```python
from build123d import *

# Parameters (mm, degrees)
ESBO_O1_W                  = 42.2
ESBO_O1_H                  = 42.2
RESSALTO_EXTRUS_O1_DEPTH   = 16
CHANFRO4_SIZE              = 7
FILETE3_R                  = 4
ESBO_O2_W                  = 42.3
ESBO_O2_H                  = 42.3
RESSALTO_EXTRUS_O2_DEPTH   = 8
CHANFRO5_SIZE              = 7
FILETE4_R                  = 4
CHANFRO5_OF_ESPELHAR1_SIZE = 7
FILETE4_OF_ESPELHAR1_R     = 4
ESBO_O3_R                  = 11
ESBO_O3_R_2                = 3.5
RESSALTO_EXTRUS_O3_DEPTH   = 2
FILETE5_R                  = 0.5
FILETE6_R                  = 1
ESBO_O4_R                  = 1.5
CORTE_EXTRUS_O1_DEPTH      = 10
PADR_OCIRCULAR1_COUNT      = 4
ESBO_O5_R                  = 2.5
RESSALTO_EXTRUS_O4_DEPTH   = 4
RESSALTO_EXTRUS_O5_DEPTH   = 19
CHANFRO3_SIZE              = 0.5
FILETE2_R                  = 0.5


with BuildPart() as part:
    # Esboço1 → Ressalto-extrusão1 (new, symmetric)
    with BuildSketch(Plane(origin=(0, 0, 0), x_dir=(1, 0, 0), z_dir=(0, 1, 0))):
        Rectangle(ESBO_O1_W, ESBO_O1_H)
    extrude(amount=RESSALTO_EXTRUS_O1_DEPTH, both=True)

    # Chanfro4
    chanfro4_edges = [part.edges().sort_by_distance(p)[0] for p in [
        (21.1, 0, 21.1),
        (-21.1, 0, 21.1),
        (-21.1, 0, -21.1),
        (21.1, 0, -21.1),
    ]]
    chamfer(chanfro4_edges, length=CHANFRO4_SIZE)

    # Filete3
    filete3_edges = [part.edges().sort_by_distance(p)[0] for p in [
        (14.1, 0, 21.1),
        (-14.1, 0, 21.1),
        (-21.1, 0, -14.1),
        (-21.1, 0, 14.1),
        (14.1, 0, -21.1),
        (-14.1, 0, -21.1),
        (21.1, 0, 14.1),
        (21.1, 0, -14.1),
    ]]
    fillet(filete3_edges, radius=FILETE3_R)

    # Esboço2 → Ressalto-extrusão2 (add)
    with BuildSketch(Plane(origin=(0, 16, 0), x_dir=(1, 0, 0), z_dir=(0, 1, 0))):
        Rectangle(ESBO_O2_W, ESBO_O2_H)
    ressalto_extrus_o2 = extrude(amount=RESSALTO_EXTRUS_O2_DEPTH)

    # Chanfro5
    chanfro5_edges = [part.edges().sort_by_distance(p)[0] for p in [
        (21.15, 20, 21.15),
        (21.15, 20, -21.15),
        (-21.15, 20, -21.15),
        (-21.15, 20, 21.15),
    ]]
    chamfer(chanfro5_edges, length=CHANFRO5_SIZE)

    # Filete4
    filete4_edges = [part.edges().sort_by_distance(p)[0] for p in [
        (-14.15, 20, -21.15),
        (14.15, 20, -21.15),
        (21.15, 20, 14.15),
        (21.15, 20, -14.15),
        (-14.15, 20, 21.15),
        (14.15, 20, 21.15),
        (-21.15, 20, -14.15),
        (-21.15, 20, 14.15),
    ]]
    fillet(filete4_edges, radius=FILETE4_R)

    # Espelhar1: Ressalto-extrusão2 across plane
    add(ressalto_extrus_o2.mirror(Plane.ZX))

    # Chanfro5 of Espelhar1
    chanfro5_of_espelhar1_edges = [part.edges().sort_by_distance(p)[0] for p in [
        (21.15, -20, 21.15),
        (21.15, -20, -21.15),
        (-21.15, -20, -21.15),
        (-21.15, -20, 21.15),
    ]]
    chamfer(chanfro5_of_espelhar1_edges, length=CHANFRO5_OF_ESPELHAR1_SIZE)

    # Filete4 of Espelhar1
    filete4_of_espelhar1_edges = [part.edges().sort_by_distance(p)[0] for p in [
        (-14.15, -20, -21.15),
        (14.15, -20, -21.15),
        (21.15, -20, 14.15),
        (21.15, -20, -14.15),
        (-14.15, -20, 21.15),
        (14.15, -20, 21.15),
        (-21.15, -20, -14.15),
        (-21.15, -20, 14.15),
    ]]
    fillet(filete4_of_espelhar1_edges, radius=FILETE4_OF_ESPELHAR1_R)

    # Esboço3 → Ressalto-extrusão3 (add)
    with BuildSketch(Plane(origin=(0, 24, 0), x_dir=(1, 0, 0), z_dir=(0, 1, 0))):
        with Locations(Location((0, 0, 0), (0, 0, 270))):
            Circle(ESBO_O3_R)
        with Locations(Location((0, 0, 0), (0, 0, 270))):
            Circle(ESBO_O3_R_2, mode=Mode.SUBTRACT)
    extrude(amount=RESSALTO_EXTRUS_O3_DEPTH)

    # Filete5
    filete5_edges = [part.edges().sort_by_distance(p)[0] for p in [
        (0, 26, -11),
    ]]
    fillet(filete5_edges, radius=FILETE5_R)

    # Filete6
    filete6_edges = [part.edges().sort_by_distance(p)[0] for p in [
        (0, 24, -11),
    ]]
    fillet(filete6_edges, radius=FILETE6_R)

    # Esboço4 → Corte-extrusão1 (cut)
    with BuildSketch(Plane(origin=(0, 24, 0), x_dir=(1, 0, 0), z_dir=(0, 1, 0))):
        with Locations(Location((-15.5, 15.5, 0), (0, 0, 270))):
            Circle(ESBO_O4_R)
    corte_extrus_o1 = extrude(amount=-CORTE_EXTRUS_O1_DEPTH, mode=Mode.SUBTRACT)

    # PadrãoCircular1: Corte-extrusão1 ×4 about axis
    padr_ocircular1_axis = Axis((0, 0, 0), (0, 1, 0))
    for i in range(1, PADR_OCIRCULAR1_COUNT):
        add(corte_extrus_o1.rotate(padr_ocircular1_axis, i * 360 / PADR_OCIRCULAR1_COUNT), mode=Mode.SUBTRACT)

    # Esboço5 → Ressalto-extrusão4 (add)
    with BuildSketch(Plane(origin=(0, 24, 0), x_dir=(1, 0, 0), z_dir=(0, 1, 0))):
        with Locations(Location((0, 0, 0), (0, 0, 270))):
            Circle(ESBO_O5_R)
    extrude(amount=RESSALTO_EXTRUS_O4_DEPTH)

    # Esboço6 → Ressalto-extrusão5 (add)
    with BuildSketch(Plane(origin=(0, 28, 0), x_dir=(1, 0, 0), z_dir=(0, 1, 0))):
        with BuildLine():
            ThreePointArc((2.5, 0), (-1.118033989, 2.236067977), (-1.5, -2))
            Line((-1.5, -2), (1.5, -2))
            ThreePointArc((1.5, -2), (2.236067977, -1.118033989), (2.5, 0))
        make_face()
    extrude(amount=RESSALTO_EXTRUS_O5_DEPTH)

    # Chanfro3
    chanfro3_edges = [part.edges().sort_by_distance(p)[0] for p in [
        (0, 47, -2.5),
    ]]
    chamfer(chanfro3_edges, length=CHANFRO3_SIZE - 0.0001)  # a hair under: the kernel refuses the full size

    # Filete2
    filete2_edges = [part.edges().sort_by_distance(p)[0] for p in [
        (-1.5, 37.25005, 2),
        (1.5, 37.25005, 2),
    ]]
    fillet(filete2_edges, radius=FILETE2_R)


solid = part.part
```
Source: CAD feature listing. Evaluate the final solid. Frame: model axes, mm. A direction names the side the tool comes from. Give positions to 0.01 mm unless a question says otherwise; leave off trailing zeros. Order: outer loops, then holes, each group sorted by start corner. A loop starts at its lowest first (then second) coordinate and runs counter-clockwise, first axis right, second up. Notation, with made-up numbers: (-37, -26) -> (-21, -26) arc R21 ccw to (-21, 0) -> close; hole circle Ø10 at (23.25, 47.5). An arc over 180 degrees is marked (long way). Use a Markdown table: item, result.
Q1. Material intervals for line 1 (X direction, y = 24.9, z = 0); line 2 (X direction, y = 20, z = 15); line 3 (Z direction, x = 15.5, y = 21.25), sorted ascending. Write a range as [from, to].
A:
| item | result |
|---|---|
| line 1 | [-11.01, -3.5], [-2.5, 2.5], [3.5, 11.01] |
| line 2 | [-20.27, -16.91], [-14.09, 14.09], [16.91, 20.27] |
| line 3 | [-19.8, -17], [-14, 14], [17, 19.8] |
Q2. Access query for faces 1 (the face through (0, 37, 2)), 2 (the face through (13.954, 0.224, 20.804)), 3 (the face through (-10.74, 25.25, -2.38)). Directions: +Z, -Z, +X, -X, +Y, -Y. A direction counts if a zero-diameter tool reaches every point of the face in a straight line with its end or side. Return the directions, or none.
A:
| item | result |
|---|---|
| face 1 | +Z, +X, -X, +Y |
| face 2 | +Z, +X |
| face 3 | +Y |
Q3. Pull-direction query (Y, two-part tool) for faces 4 (the face through (-20.854, 20.056, 14.004)), 5 (the face through (-20.804, 0.224, 13.954)), 6 (the face through (-16, 14, 15)); classes: +Y half, -Y half, draft (parallel to the pull), parting line (faces both ways), or undercut.
A:
| item | result |
|---|---|
| face 4 | draft |
| face 5 | undercut |
| face 6 | +Y half |
Q4. First-contact query: P1, Ø12.5, axis at x = 5.5, z = 4, coming from the +Y side; P2, Ø2, axis at x = -7.5, z = -9, coming from the +Y side; P3, Ø3.5, axis at x = 15, z = -15.5, coming from the +Y side; P4, Ø1, axis at x = 6.5, y = 3.5, coming from the -Z side. Flat tips, straight axial feed; report the tip coordinate or a pass-through.
A:
| item | result |
|---|---|
| P1 | y = 47 |
| P2 | y = 25.95 |
| P3 | y = 24 |
| P4 | z = -21.1 |
Q5. Section A-A (y = -11.5). Return the cut outline in (x, z).
A:
| item | result |
|---|---|
| outline | (-21.1, -12.44) arc R4 ccw to (-19.93, -15.27) -> (-15.27, -19.93) arc R4 ccw to (-12.44, -21.1) -> (12.44, -21.1) arc R4 ccw to (15.27, -19.93) -> (19.93, -15.27) arc R4 ccw to (21.1, -12.44) -> (21.1, 12.44) arc R4 ccw to (19.93, 15.27) -> (15.27, 19.93) arc R4 ccw to (12.44, 21.1) -> (-12.44, 21.1) arc R4 ccw to (-15.27, 19.93) -> (-19.93, 15.27) arc R4 ccw to (-21.1, 12.44) -> close |
